For this review, take the finished solid that the model builds, in its own axes (mm). Face numbers are marked on the shaded views. Round coordinates to 2 decimals unless told otherwise and drop trailing zeros. Order: outer loops, then holes, each group sorted by start corner. A loop starts at its lowest first (then second) coordinate and runs counter-clockwise, first axis right, second up. Notation, with made-up numbers: M -36.75,-23 L 18.25,-23 A28 cw 18.25,6 Z; hole C 37.5,69 d10. An arc over 180 degrees is marked long. Write item = value, one per line. Start each with the question number.
from build123d import *

# Parameters (mm, degrees)
BOSS_EXTRUDE1_DEPTH = 1.524
SKETCH2_W           = 9.144
SKETCH2_H           = 7.62
BOSS_EXTRUDE2_DEPTH = 4.064
SKETCH3_W           = 5.08
SKETCH3_H           = 7.874
BOSS_EXTRUDE3_DEPTH = 5.08
SKETCH4_W           = 20.32
SKETCH4_H           = 2.54
BOSS_EXTRUDE4_DEPTH = 3.81
SKETCH6_W           = 6.858
SKETCH6_H           = 3.302
BOSS_EXTRUDE5_DEPTH = 2.286
SKETCH7_W           = 1.27
SKETCH7_H           = 0.762
BOSS_EXTRUDE6_DEPTH = 0.889


with BuildPart() as part:
    # Sketch1 → Boss-Extrude1 (new body)
    with BuildSketch(Plane.XY):
        Polygon((-10.536438109, -12.7), (32.389561792, -12.7), (32.389561792, 12.7), (-10.536438109, 12.7), (-12.060438109, 14.224), (-32.380438109, 14.224), (-32.380438109, -14.224), (-12.060438109, -14.224), align=None)
    extrude(amount=BOSS_EXTRUDE1_DEPTH)

    # Sketch2 → Boss-Extrude2 (add)
    with BuildSketch(Plane.XY.offset(1.524)):
        with Locations((-28.316438109, -4.826)):
            Rectangle(SKETCH2_W, SKETCH2_H)
    extrude(amount=BOSS_EXTRUDE2_DEPTH)

    # Sketch3 → Boss-Extrude3 (add)
    with BuildSketch(Plane.XY.offset(1.524)):
        with Locations((-28.570438109, 5.207)):
            Rectangle(SKETCH3_W, SKETCH3_H)
    extrude(amount=BOSS_EXTRUDE3_DEPTH)

    # Sketch4 → Boss-Extrude4 (add)
    with BuildSketch(Plane(origin=(0, 0, 0), x_dir=(-1, 0, 0), z_dir=(0, 0, -1))):
        with Locations((21.712438109, 11.049)):
            Rectangle(SKETCH4_W, SKETCH4_H)
    boss_extrude4 = extrude(amount=BOSS_EXTRUDE4_DEPTH)

    # Mirror1: Boss-Extrude4 across plane
    add(boss_extrude4.mirror(Plane.ZX))

    # Sketch6 → Boss-Extrude5 (add)
    with BuildSketch(Plane.XY.offset(1.524)):
        with Locations((-7.361438109, 9.271)):
            Rectangle(SKETCH6_W, SKETCH6_H)
    extrude(amount=BOSS_EXTRUDE5_DEPTH)

    # Sketch7 → Boss-Extrude6 (add)
    with BuildSketch(Plane.XY.offset(3.81)):
        with Locations((-6.853438109, 10.541)):
            Rectangle(SKETCH7_W, SKETCH7_H)
    extrude(amount=BOSS_EXTRUDE6_DEPTH)


solid = part.part
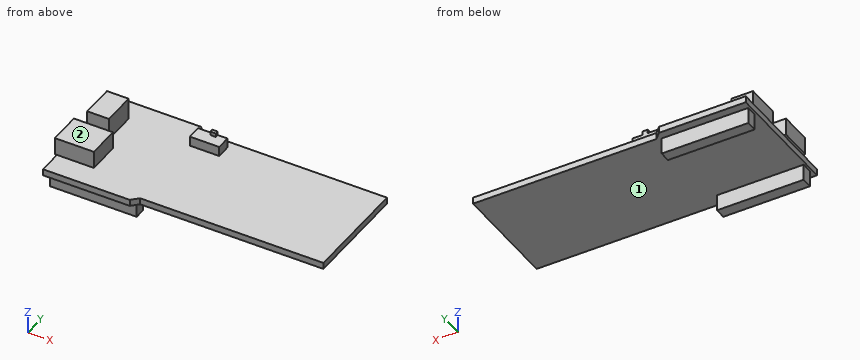
(1) We need section B-B, the plane x = -27.5. Write out the cut boundary in (y, z).
(2) We need section D-D, the plane z = 2.5. Write out the cut boundary in (x, y).
(3) For line 1 along Y through (x, z) = (-26.5, -0.25); line 2 along X through (y, z) = (-3.5, 5); line 3 along Z through (x, y) = (-29.5, 11.75), list the stretches that pass through material, from the lowest coordinate up.
(4) Draft analysis for pull direction Y (two halves, no side actions). For the marked faces 1 and 2, state which applies: released by +Y, released by -Y, zero draft, split by the parting line, or undercut.
(5) We need section A-A, the plane z = -3. Write out the cut boundary in (x, y), then the cut area to 3 significant figures.
(6) Insertion check: pin 1 (1.7 mm diameter, centred on x = 2, z = 1, fed in from +Y); pin 2 (1.8 mm diameter, centred on y = 9, z = 3, fed in from +X); pin 3 (1.3 mm diameter, centred on y = 10.5, z = -1.5, fed in from +X); pin 4 (1 mm diameter, centred on x = 17, z = -1.5, fed in from -Y). Each pin has a flat end and moves straight along its axis. Give the tip position at first contact, or say it passes through.
(7) We need section C-C, the plane y = 8.5. Write out the cut boundary in (x, z), then the cut area to 3 significant figures.
Values:
q1.outline = M -14.22,0 L -12.32,0 L -12.32,-3.81 L -9.78,-3.81 L -9.78,0 L 9.78,0 L 9.78,-3.81 L 12.32,-3.81 L 12.32,0 L 14.22,0 L 14.22,1.52 L 9.14,1.52 L 9.14,6.6 L 1.27,6.6 L 1.27,1.52 L -1.02,1.52 L -1.02,5.59 L -8.64,5.59 L -8.64,1.52 L -14.22,1.52 Z
q2.outline = M -32.89,-8.64 L -23.74,-8.64 L -23.74,-1.02 L -32.89,-1.02 Z; M -31.11,1.27 L -26.03,1.27 L -26.03,9.14 L -31.11,9.14 Z; M -10.79,7.62 L -3.93,7.62 L -3.93,10.92 L -10.79,10.92 Z
q3.line_1 = -12.32 to -9.78, 9.78 to 12.32
q3.line_2 = -32.89 to -23.74
q3.line_3 = -3.81 to 1.52
q4.face_1 = undercut
q4.face_2 = zero draft
q5.outline = M -31.87,-12.32 L -11.55,-12.32 L -11.55,-9.78 L -31.87,-9.78 Z; M -31.87,9.78 L -11.55,9.78 L -11.55,12.32 L -31.87,12.32 Z
q5.area = 103 mm²
q6.pin_1 = 12.7
q6.pin_2 = -3.93
q6.pin_3 = -11.55
q6.pin_4 = through
q7.outline = M -32.38,0 L 32.39,0 L 32.39,1.52 L -3.93,1.52 L -3.93,3.81 L -10.79,3.81 L -10.79,1.52 L -26.03,1.52 L -26.03,6.6 L -31.11,6.6 L -31.11,1.52 L -32.38,1.52 Z
q7.area = 140 mm²
